Work out the finished part from the listing and answer in its coordinate system (mm). Face numbers are marked on the shaded views. A direction names the side the tool comes from. Round coordinates to 2 decimals unless told otherwise and drop trailing zeros. Write each loop counter-clockwise with the first axis right and the second up, starting at its lowest first coordinate (ties: lowest second). Pieces come first, ordered by that corner, then holes. Notation, with made-up numbers: M 43.25,61 L 70.25,61 A17 ccw 70.25,66 Z; hole C 59,39 d1. An arc over 180 degrees is marked long. One line per item, written item: value. Start each with the question number.
Q1. A tool of negligible diameter and unlimited length cuts with its end or side. For the marked faces 1 and 2, from which of +Z, -Z, +X, -X, +Y, -Y can it reach the whole face along a straight path? Write none if from no direction.
Q2. Find section C-C (y = -0.75). Write down the section's boundary in (x, z), and give its area (3 significant figures).
Q3. Given pin 1 Ø2 at (y, z) = (-1.5, 2) entering from +X; pin 2 Ø2 at (x, z) = (-5, -2) entering from -Y; pin 3 Ø2 at (y, z) = (-3.5, -2) entering from -X, each flat-ended and moving along its own axis, determine where each tip first touches the part or whether it passes through.
Q4. Consider probe 1 along Y at (x, z) = (3, -2.5); probe 2 along Z at (x, y) = (0, -2.25); probe 3 along X at (y, z) = (0.75, 1). Determine where each line is inside the solid, lowest interval first.
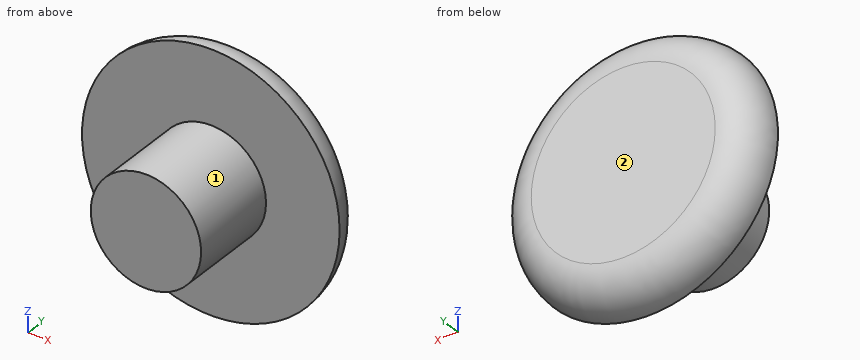
from build123d import *

# Parameters (mm, degrees)
F0_R     = 3
F1_DEPTH = 5
F0_R_2   = 7
F2_DEPTH = 2
F3_R     = 1.99999


# Not quite as in the source:
# - a fillet or chamfer is up to 0.001 mm smaller than in the source, because OpenCascade refuses the exact size


with BuildPart() as f1:
    # F0 (on Front) → F1 (new body)
    with BuildSketch(Plane.XZ):
        Circle(F0_R)
    extrude(amount=F1_DEPTH)

    # F0 (on Front) → F2 (join)
    with BuildSketch(Plane.XZ):
        Circle(F0_R_2)
        Circle(F0_R, mode=Mode.SUBTRACT)
        Circle(F0_R)
    extrude(amount=-F2_DEPTH)

    # F3 (radius 2 in the source; OpenCascade refuses exactly that, so slightly less here)
    f3_edges = [f1.edges().sort_by_distance(p)[0] for p in [
        (-7, 2, 0),
    ]]
    fillet(f3_edges, radius=F3_R)


solid = f1.part
The answers:
1. face 1: -Y
1. face 2: +Z, -Z, +X, -X, +Y
2. outline: C 0,0 d6
2. area: 28.3 mm2
3. pin 1: x = 2.83
3. pin 2: y = 0
3. pin 3: x = -2.83
4. probe 1: 0 to 2
4. probe 2: -3 to 3
4. probe 3: -6.78 to 6.78
